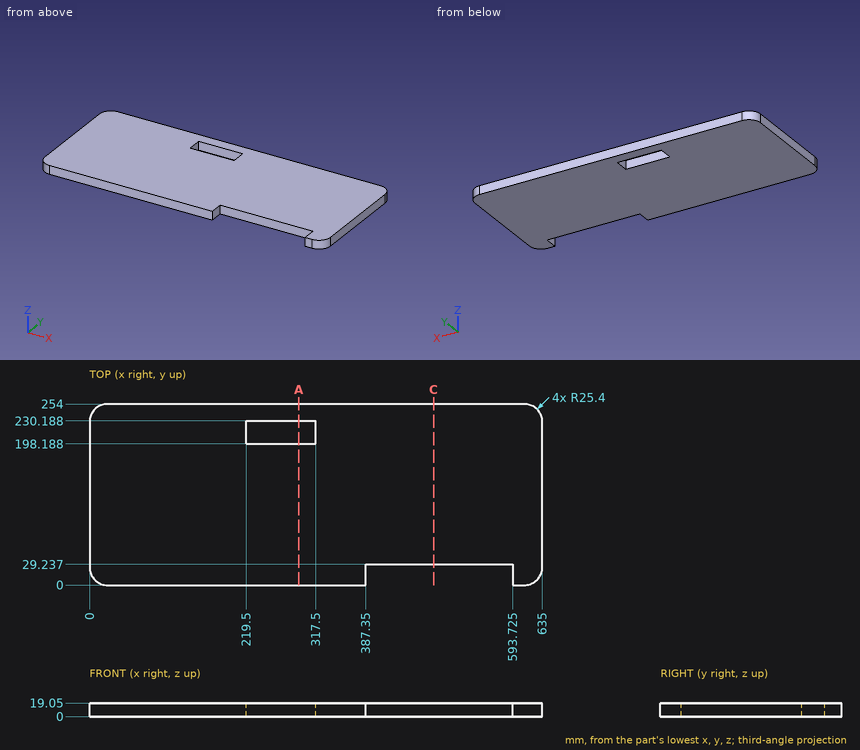
Answer from the drawing. Dimensions are ordinates in mm from the lowest x, y and z of the part. Give positions to 0.01 mm unless a question says otherwise; leave off trailing zeros. Write each loop counter-clockwise with the first axis right and the second up, starting at its lowest first coordinate (ties: lowest second). Pieces come first, ordered by that corner, then holes. Notation, with made-up numbers: (28, -28.75) - (86, -28.75) arc R15 cw to (86, -12.75) - close; hole circle Ø1 at (-20, 48). An arc over 180 degrees is marked (long way). One line per item, written item: value. Start each with the question number.
1. Consider probe 1 along X at (y, z) = (201, 13.5); probe 2 along Y at (x, z) = (244, 15.25); probe 3 along Y at (x, z) = (459, 8.5). Determine where each line is inside the solid, lowest interval first.
2. Find section C-C (x = 482.5). Write down the section's boundary in (y, z).
3. Find section A-A (x = 293.5). Write down the section's boundary in (y, z).
Geometry results:
1. probe 1: 0 to 219.5, 317.5 to 635
1. probe 2: 0 to 198.19, 230.19 to 254
1. probe 3: 29.24 to 254
2. outline: (29.24, 0) - (254, 0) - (254, 19.05) - (29.24, 19.05) - close
3. outline: (0, 0) - (198.19, 0) - (198.19, 19.05) - (0, 19.05) - close; (230.19, 0) - (254, 0) - (254, 19.05) - (230.19, 19.05) - close
